from build123d import *

# Parameters (mm, degrees)
BOSS_EXTRUDE1_DEPTH     = 55
SHELL1_START            = 3
SHELL1_DEPTH            = 49
CUT_EXTRUDE1_DEPTH      = 161.15617378
CUT_EXTRUDE1_DEPTH_BACK = 161.15617378
SKETCH4_W               = 154.651671352
SKETCH4_H               = 22.597591031
SKETCH6_R               = 3.8
BOSS_EXTRUDE2_DEPTH     = 6
BOSS_EXTRUDE3_DEPTH     = 37
SKETCH9_W               = 26
SKETCH9_H               = 10
BOSS_EXTRUDE4_DEPTH     = 5
CUT_EXTRUDE3_REACH      = 159.293
SKETCH10_R              = 1.75
SKETCH11_W              = 26
SKETCH11_H              = 2
SKETCH11_W_2            = 11.5
SKETCH11_H_2            = 7.1
BOSS_EXTRUDE5_DEPTH     = 5
CUT_EXTRUDE4_REACH      = 184.818
SKETCH12_W              = 15
SKETCH12_H              = 10
SKETCH13_W              = 20
SKETCH13_H              = 40.9
BOSS_EXTRUDE6_DEPTH     = 11.5
CUT_EXTRUDE5_DEPTH      = 11.5
BOSS_EXTRUDE7_DEPTH     = 11.5
CUT_EXTRUDE6_REACH      = 158.036
SKETCH16_W              = 15
SKETCH16_H              = 10
BOSS_EXTRUDE8_DEPTH     = 37
BOSS_EXTRUDE9_DEPTH     = 5
SKETCH20_W              = 40.9
SKETCH20_H              = 20
BOSS_EXTRUDE10_DEPTH    = 11.5
CUT_EXTRUDE7_DEPTH      = 11.5


# Read off the part's stored shape, not the designer's step: Shell1
with BuildPart() as part:
    # Sketch2 → Boss-Extrude1 (new body)
    with BuildSketch(Plane(origin=(0, 0, 0), x_dir=(1, 0, 0), z_dir=(0, 1, 0))):
        Polygon((9, 55), (0, 46), (0, 9), (9, 0), (85, 0), (140, 0), (140, 46), (131, 55), align=None)
        Polygon((140, 0), (85, 0), (85, -46), (94, -55), (131, -55), (140, -46), align=None)
    extrude(amount=BOSS_EXTRUDE1_DEPTH)

    # Shell1 outline → Shell1 (cut)
    with BuildSketch(Plane(origin=(0, 0, 0), x_dir=(1, 0, 0), z_dir=(0, 1, 0)).offset(SHELL1_START)):
        Polygon((10.242640687, 3), (88, 3), (88, -44.757359313), (95.242640687, -52), (129.757359313, -52), (137, -44.757359313), (137, 44.757359313), (129.757359313, 52), (10.242640687, 52), (3, 44.757359313), (3, 10.242640687), align=None)
    extrude(amount=SHELL1_DEPTH, mode=Mode.SUBTRACT)

    # Sketch4 → Cut-Extrude1 (cut, two sides: drawn at the far end of the back side and taken through both)
    with BuildSketch(Plane.XY.offset(-CUT_EXTRUDE1_DEPTH_BACK)):
        with Locations((70, 52.798795516)):
            Rectangle(SKETCH4_W, SKETCH4_H)
    extrude(amount=CUT_EXTRUDE1_DEPTH + CUT_EXTRUDE1_DEPTH_BACK, mode=Mode.SUBTRACT)

    # Sketch6 → Boss-Extrude2 (add)
    with BuildSketch(Plane.XZ):
        with Locations(Location((112.5, 30, 0), (0, 0, 270))):
            Circle(SKETCH6_R)
    extrude(amount=BOSS_EXTRUDE2_DEPTH)

    # Sketch8 → Boss-Extrude3 (add)
    with BuildSketch(Plane(origin=(0, 3, 0), x_dir=(1, 0, 0), z_dir=(0, 1, 0))):
        Polygon((102.5, -35), (99.5, -35), (99.5, -43), (104.5, -43), (104.5, -40), (102.5, -40), align=None)
        Polygon((99.5, 3.9), (99.5, -4.1), (102.5, -4.1), (102.5, 0.9), (104.5, 0.9), (104.5, 3.9), align=None)
        Polygon((120.5, -40), (120.5, -43), (125.5, -43), (125.5, -35), (122.5, -35), (122.5, -40), align=None)
        Polygon((125.5, 3.9), (120.5, 3.9), (120.5, 0.9), (122.5, 0.9), (122.5, -4.1), (125.5, -4.1), align=None)
    extrude(amount=BOSS_EXTRUDE3_DEPTH)

    # Sketch9 → Boss-Extrude4 (add)
    with BuildSketch(Plane(origin=(0, 40, 0), x_dir=(1, 0, 0), z_dir=(0, 1, 0))):
        with Locations((112.5, 5.9)):
            Rectangle(SKETCH9_W, SKETCH9_H)
        with Locations((112.5, -45)):
            Rectangle(SKETCH9_W, SKETCH9_H)
    extrude(amount=-BOSS_EXTRUDE4_DEPTH)

    # Sketch10 → Cut-Extrude3 (cut, up to next)
    with BuildSketch(Plane(origin=(0, 40, 0), x_dir=(1, 0, 0), z_dir=(0, 1, 0)), mode=Mode.PRIVATE) as cut_extrude3_sk1:
        with Locations(Location((107.5, 4.5, 0), (0, 0, 270))):
            Circle(SKETCH10_R)
    cut_extrude3_tool1 = extrude(cut_extrude3_sk1.sketch, amount=-CUT_EXTRUDE3_REACH, mode=Mode.PRIVATE) & part.part
    # Sketch10 → Cut-Extrude3 (cut, up to next)
    with BuildSketch(Plane(origin=(0, 40, 0), x_dir=(1, 0, 0), z_dir=(0, 1, 0)), mode=Mode.PRIVATE) as cut_extrude3_sk2:
        with Locations(Location((117.5, 4.5, 0), (0, 0, 270))):
            Circle(SKETCH10_R)
    cut_extrude3_tool2 = extrude(cut_extrude3_sk2.sketch, amount=-CUT_EXTRUDE3_REACH, mode=Mode.PRIVATE) & part.part
    # Sketch10 → Cut-Extrude3 (cut, up to next)
    with BuildSketch(Plane(origin=(0, 40, 0), x_dir=(1, 0, 0), z_dir=(0, 1, 0)), mode=Mode.PRIVATE) as cut_extrude3_sk3:
        with Locations(Location((117.5, -43.6, 0), (0, 0, 270))):
            Circle(SKETCH10_R)
    cut_extrude3_tool3 = extrude(cut_extrude3_sk3.sketch, amount=-CUT_EXTRUDE3_REACH, mode=Mode.PRIVATE) & part.part
    # Sketch10 → Cut-Extrude3 (cut, up to next)
    with BuildSketch(Plane(origin=(0, 40, 0), x_dir=(1, 0, 0), z_dir=(0, 1, 0)), mode=Mode.PRIVATE) as cut_extrude3_sk4:
        with Locations(Location((107.5, -43.6, 0), (0, 0, 90))):
            Circle(SKETCH10_R)
    cut_extrude3_tool4 = extrude(cut_extrude3_sk4.sketch, amount=-CUT_EXTRUDE3_REACH, mode=Mode.PRIVATE) & part.part
    add(cut_extrude3_tool1.solids().sort_by_distance((107.5, 40, -4.5))[0], mode=Mode.SUBTRACT)
    add(cut_extrude3_tool2.solids().sort_by_distance((117.5, 40, -4.5))[0], mode=Mode.SUBTRACT)
    add(cut_extrude3_tool3.solids().sort_by_distance((117.5, 40, 43.6))[0], mode=Mode.SUBTRACT)
    add(cut_extrude3_tool4.solids().sort_by_distance((107.5, 40, 43.6))[0], mode=Mode.SUBTRACT)

    # Sketch11 → Boss-Extrude5 (add)
    with BuildSketch(Plane(origin=(0, 40, 0), x_dir=(1, 0, 0), z_dir=(0, 1, 0))):
        with Locations((112.5, -51)):
            Rectangle(SKETCH11_W, SKETCH11_H)
        with Locations((93.75, -0.55)):
            Rectangle(SKETCH11_W_2, SKETCH11_H_2)
        with Locations((131.25, -0.55)):
            Rectangle(SKETCH11_W_2, SKETCH11_H_2)
    extrude(amount=-BOSS_EXTRUDE5_DEPTH)

    # Sketch12 → Cut-Extrude4 (cut, up to next)
    with BuildSketch(Plane.XY.offset(55), mode=Mode.PRIVATE) as cut_extrude4_sk1:
        with Locations((112.5, 20)):
            Rectangle(SKETCH12_W, SKETCH12_H)
    cut_extrude4_tool1 = extrude(cut_extrude4_sk1.sketch, amount=-CUT_EXTRUDE4_REACH, mode=Mode.PRIVATE) & part.part
    add(cut_extrude4_tool1.solids().sort_by_distance((112.5, 20, 55))[0], mode=Mode.SUBTRACT)

    # Sketch13 → Boss-Extrude6 (add)
    with BuildSketch(Plane(origin=(0, 3, 0), x_dir=(1, 0, 0), z_dir=(0, 1, 0))):
        with Locations((112.5, -19.55)):
            Rectangle(SKETCH13_W, SKETCH13_H)
    extrude(amount=BOSS_EXTRUDE6_DEPTH)

    # Sketch14 → Cut-Extrude5 (cut)
    with BuildSketch(Plane(origin=(0, 14.5, 0), x_dir=(1, 0, 0), z_dir=(0, 1, 0))):
        Polygon((105.5, -2.1), (105.5, -4.1), (105.5, -35), (105.5, -37), (119.5, -37), (119.5, -35), (119.5, -4.1), (119.5, -2.1), align=None)
    extrude(amount=-CUT_EXTRUDE5_DEPTH, mode=Mode.SUBTRACT)

    # Sketch15 → Boss-Extrude7 (add)
    with BuildSketch(Plane(origin=(0, 3, 0), x_dir=(1, 0, 0), z_dir=(0, 1, 0))):
        Polygon((112.5, -19.55), (119.5, -2.1), (117.883811276, -2.1), (111.107835851, -18.991538737), align=None)
        Polygon((119.5, -6.128927606), (119.5, -2.1), (112.5, -19.55), (113.892164149, -20.108461263), align=None)
        Polygon((105.5, -37), (112.5, -19.55), (111.107835851, -18.991538737), (105.5, -32.971072394), align=None)
        Polygon((113.892164149, -20.108461263), (112.5, -19.55), (105.5, -37), (107.116188724, -37), align=None)
    extrude(amount=BOSS_EXTRUDE7_DEPTH)

    # Sketch16 → Cut-Extrude6 (cut, up to next)
    with BuildSketch(Plane.ZY, mode=Mode.PRIVATE) as cut_extrude6_sk1:
        with Locations((-27.5, 20)):
            Rectangle(SKETCH16_W, SKETCH16_H)
    cut_extrude6_tool1 = extrude(cut_extrude6_sk1.sketch, amount=-CUT_EXTRUDE6_REACH, mode=Mode.PRIVATE) & part.part
    add(cut_extrude6_tool1.solids().sort_by_distance((0, 20, -27.5))[0], mode=Mode.SUBTRACT)

    # Sketch18 → Boss-Extrude8 (add)
    with BuildSketch(Plane(origin=(0, 3, 0), x_dir=(1, 0, 0), z_dir=(0, 1, 0))):
        Polygon((15, 37.5), (20, 37.5), (20, 40.5), (12, 40.5), (12, 35.5), (15, 35.5), align=None)
        Polygon((55.9, 37.5), (55.9, 35.5), (58.9, 35.5), (58.9, 40.5), (50.9, 40.5), (50.9, 37.5), align=None)
        Polygon((55.9, 19.5), (55.9, 17.5), (50.9, 17.5), (50.9, 14.5), (58.9, 14.5), (58.9, 19.5), align=None)
        Polygon((20, 14.5), (20, 17.5), (15, 17.5), (15, 19.5), (12, 19.5), (12, 14.5), align=None)
    extrude(amount=BOSS_EXTRUDE8_DEPTH)

    # Sketch19 → Boss-Extrude9 (add)
    # profile 1 of 3: a face of its own
    with BuildSketch(Plane(origin=(0, 40, 0), x_dir=(1, 0, 0), z_dir=(0, 1, 0))):
        Polygon((12, 35.5), (12, 40.5), (5, 40.5), (5, 14.5), (12, 14.5), (12, 19.5), (15, 19.5), (15, 35.5), align=None)
        with BuildLine():
            ThreePointArc((13.15, 22.5), (10.162563133, 21.262563133), (11.4, 24.25))
            ThreePointArc((11.4, 24.25), (12.637436867, 23.737436867), (13.15, 22.5))
        make_face(mode=Mode.SUBTRACT)
        with BuildLine():
            ThreePointArc((13.15, 32.5), (12.637436867, 31.262563133), (11.4, 30.75))
            ThreePointArc((11.4, 30.75), (10.162563133, 33.737436867), (13.15, 32.5))
        make_face(mode=Mode.SUBTRACT)
    # profile 2 of 3: a face of its own
    with BuildSketch(Plane(origin=(0, 40, 0), x_dir=(1, 0, 0), z_dir=(0, 1, 0))):
        Polygon((15, 37.5), (15, 40.5), (12, 40.5), (12, 35.5), (15, 35.5), align=None)
    # profile 3 of 3: a face of its own
    with BuildSketch(Plane(origin=(0, 40, 0), x_dir=(1, 0, 0), z_dir=(0, 1, 0))):
        Polygon((58.9, 19.5), (58.9, 14.5), (65.9, 14.5), (65.9, 40.5), (58.9, 40.5), (58.9, 35.5), (55.9, 35.5), (55.9, 19.5), align=None)
        with BuildLine():
            ThreePointArc((61.25, 22.5), (58.262563133, 21.262563133), (59.5, 24.25))
            ThreePointArc((59.5, 24.25), (60.737436867, 23.737436867), (61.25, 22.5))
        make_face(mode=Mode.SUBTRACT)
        with BuildLine():
            ThreePointArc((61.25, 32.5), (60.737436867, 31.262563133), (59.5, 30.75))
            ThreePointArc((59.5, 30.75), (58.262563133, 33.737436867), (61.25, 32.5))
        make_face(mode=Mode.SUBTRACT)
    extrude(amount=-BOSS_EXTRUDE9_DEPTH)

    # Sketch20 → Boss-Extrude10 (add)
    with BuildSketch(Plane(origin=(0, 3, 0), x_dir=(1, 0, 0), z_dir=(0, 1, 0))):
        with Locations((35.45, 27.5)):
            Rectangle(SKETCH20_W, SKETCH20_H)
    extrude(amount=BOSS_EXTRUDE10_DEPTH)

    # Sketch21 → Cut-Extrude7 (cut)
    with BuildSketch(Plane(origin=(0, 14.5, 0), x_dir=(1, 0, 0), z_dir=(0, 1, 0))):
        Polygon((18, 32.883811276), (18, 20.5), (48.871072394, 20.5), (34.891538737, 26.107835851), align=None)
        Polygon((52.9, 34.5), (22.028927606, 34.5), (36.008461263, 28.892164149), (52.9, 22.116188724), align=None)
    extrude(amount=-CUT_EXTRUDE7_DEPTH, mode=Mode.SUBTRACT)


solid = part.part
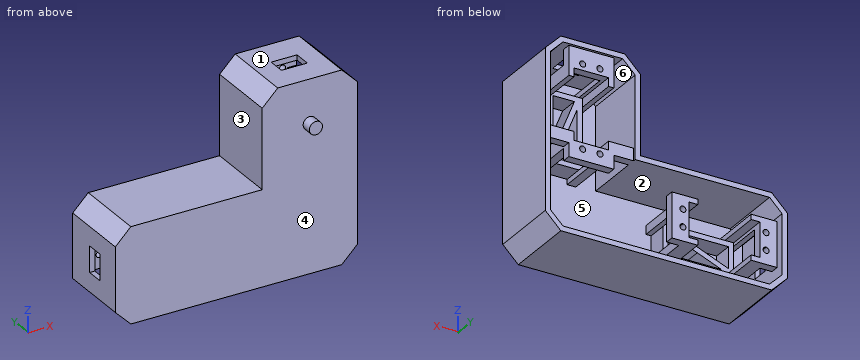
Can you work these out from the model? Positions are in its coordinate system, mm. Face numbers are marked on the shaded views. A direction names the side the tool comes from. Coordinates: 2 decimals unless noted, no trailing zeros. Write each loop counter-clockwise with the first axis right and the second up, starting at its lowest first coordinate (ties: lowest second). Pieces come first, ordered by that corner, then holes. Notation, with made-up numbers: (56, -28.75) -> (89, -28.75) arc R17 ccw to (89, -1.75) -> close; hole circle Ø5 at (13.25, 20). An arc over 180 degrees is marked (long way). Write each question's results on one line, items separated by ' | '. Start each with the question number.
Q1. If I drill on probe 1 along Z at (x, y) = (117.5, 36.2); probe 2 along X at (y, z) = (38.1, -22.5); probe 3 along X at (y, z) = (38.3, 43.6), over which ranges is the centre line in solid material (lowest first)?
Q2. On a 3-axis mill with a long thin cutter (end or side, diameter ignored), from which of +Z, -Z, +X, -X, +Y, -Y can I reach the whole of each face in a straight line? I mean the marked faces 1, 2 and 3. Say none if no direction works.
Q3. Imagine slicing it at A-A (y = 13). State how many separate pieces and enclosed holes the cut face has, then the cut area to 3 significant figures.
Q4. Imagine slicing it at C-C (z = 48.5). Write out the boundary of the cut face in (x, y), then the cut area to 3 significant figures.
Q5. I'm going to push flat-ended pins straight in: pin 1 (3.5 mm diameter, centred on x = 13.5, y = 12, fed in from +Z); pin 2 (1.5 mm diameter, centred on y = 22, z = 2, fed in from -X); pin 3 (4 mm diameter, centred on x = 107.5, z = 43.6, fed in from +Y); pin 4 (8 mm diameter, centred on x = 91, z = 1.5, fed in from +Y). Where does each tip first touch, or does it pass through?
Q6. We'd pull the mould along Y, two halves only. Please class the marked faces 4, 5 and 6: +Y half, -Y half, draft (parallel to the pull), parting line (faces both ways), or undercut.
Q7. Imagine slicing it at D-D (x = 26). Write out the boundary of the cut face in (y, z).
Taken from the geometry:
1) probe 1: z = -55 to -52, -10.9 to -6.25, -2.75 to -0.9, 40 to 41.85, 45.35 to 55 | probe 2: x = 0 to 3, 5 to 9.65, 13.15 to 15, 55.9 to 57.75, 61.25 to 65.9, 137 to 140 | probe 3: x = 85 to 88, 99.5 to 105.75, 109.25 to 115.75, 119.25 to 125.5, 137 to 140
2) face 1: +Z, +X, -X, +Y, -Y | face 2: +Y | face 3: +Z, -X, +Y, -Y
3) separate pieces: 3 | enclosed holes: 5 | area: 2,500 mm^2
4) outline: (87.5, 0) -> (137.5, 0) -> (137.5, 41.5) -> (133.26, 41.5) -> (133.26, 3) -> (91.74, 3) -> (91.74, 41.5) -> (87.5, 41.5) -> close; (99.5, 35) -> (125.5, 35) -> (125.5, 40) -> (99.5, 40) -> close | area: 607 mm^2
5) pin 1: stops at z = 0 | pin 2: stops at x = 85 | pin 3: stops at y = 40 | pin 4: stops at y = 41.5
6) face 4: -Y half | face 5: undercut | face 6: draft
7) outline: (0, -55) -> (41.5, -55) -> (41.5, -52) -> (3, -52) -> (3, -37.5) -> (14.5, -37.5) -> (14.5, -34.5) -> (3, -34.5) -> (3, -32.91) -> (14.5, -32.91) -> (14.5, -29.67) -> (3, -29.67) -> (3, -20.5) -> (14.5, -20.5) -> (14.5, -17.5) -> (3, -17.5) -> (3, -3) -> (41.5, -3) -> (41.5, 0) -> (0, 0) -> close
